Model file for the job. Use its own axes, mm. Give positions to 0.01 mm unless a question says otherwise; leave off trailing zeros. Loops run counter-clockwise (first coordinate to the right, second up) from the corner with the lowest first, then second, coordinate; pieces in that order, holes last. Notation, with made-up numbers: (72, 29) - (131, 29) arc R29 cw to (131, 61) - close; hole circle Ø8 at (-40, 66.5). An arc over 180 degrees is marked (long way). Use a Markdown table: item, result.
from build123d import *

# Parameters (mm, degrees)
SKETCH1_W               = 65.5
SKETCH1_H               = 80
BOSS_EXTRUDE1_DEPTH     = 5
SKETCH2_W               = 7.499999691
SKETCH2_H               = 80
CUT_EXTRUDE1_DEPTH      = 52.938064076
SKETCH3_R               = 12
SKETCH3_R_2             = 1.65
CUT_EXTRUDE2_DEPTH      = 52.938064076
CUT_EXTRUDE3_DEPTH      = 52.938064076
CUT_EXTRUDE3_DEPTH_BACK = 52.938064076
SKETCH4_R               = 4.025


with BuildPart() as part:
    # Sketch1 → Boss-Extrude1 (new body)
    with BuildSketch(Plane.XY):
        Rectangle(SKETCH1_W, SKETCH1_H)
    extrude(amount=BOSS_EXTRUDE1_DEPTH)

    # Sketch2 → Cut-Extrude1 (cut, through all)
    with BuildSketch(Plane.XY.offset(5)):
        with Locations((29.000000155, 0)):
            Rectangle(SKETCH2_W, SKETCH2_H)
    extrude(amount=-CUT_EXTRUDE1_DEPTH, mode=Mode.SUBTRACT)

    # Sketch3 → Cut-Extrude2 (cut, through all)
    with BuildSketch(Plane(origin=(0, 0, 0), x_dir=(-1, 0, 0), z_dir=(0, 0, -1))):
        with Locations((-1.25, 0)):
            Circle(SKETCH3_R)
        with Locations((-16.75, 15.5)):
            Circle(SKETCH3_R_2)
        with Locations((14.25, 15.5)):
            Circle(SKETCH3_R_2)
        with Locations((14.25, -15.5)):
            Circle(SKETCH3_R_2)
        with Locations((-16.75, -15.5)):
            Circle(SKETCH3_R_2)
    extrude(amount=-CUT_EXTRUDE2_DEPTH, mode=Mode.SUBTRACT)

    # Sketch4 → Cut-Extrude3 (cut, two sides: drawn at the far end of the back side and taken through both)
    with BuildSketch(Plane(origin=(0, 0, 0), x_dir=(-1, 0, 0), z_dir=(0, 0, -1)).offset(-CUT_EXTRUDE3_DEPTH_BACK)):
        with Locations((-1.25, 30)):
            Circle(SKETCH4_R)
        with Locations(Location((-1.25, -30, 0), (0, 0, 180))):
            Circle(SKETCH4_R)
    extrude(amount=CUT_EXTRUDE3_DEPTH + CUT_EXTRUDE3_DEPTH_BACK, mode=Mode.SUBTRACT)


solid = part.part
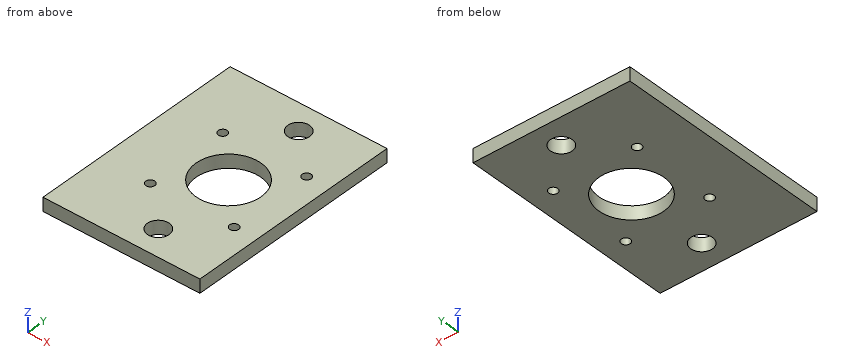
(1) Slice it at B-B, the plane y = 0. Write the cut outline in (x, z).
Computed:
| item | result |
|---|---|
| outline | (-32.75, 0) - (-10.75, 0) - (-10.75, 5) - (-32.75, 5) - close; (13.25, 0) - (25.25, 0) - (25.25, 5) - (13.25, 5) - close |
(2) Drill centre lines: probe 1 along Y at (x, z) = (-14.5, 3.75); probe 2 along Y at (x, z) = (1.25, 3.85) (3 decimals); probe 3 along X at (y, z) = (30, 2) (3 decimals). Where is each one in solid material? Low to high. Write a range as [from, to].
Computed:
| item | result |
|---|---|
| probe 1 | [-40, -17.13], [-13.87, 13.87], [17.13, 40] |
| probe 2 | [-40, -34.025], [-25.975, -12], [12, 25.975], [34.025, 40] |
| probe 3 | [-32.75, -2.775], [5.275, 25.25] |
(3) Slice it at A-A, the plane x = 1.25. Write the cut outline in (y, z) (3 decimals), plus the area to 4 significant figures.
Computed:
| item | result |
|---|---|
| outline | (-40, 0) - (-34.025, 0) - (-34.025, 5) - (-40, 5) - close; (-25.975, 0) - (-12, 0) - (-12, 5) - (-25.975, 5) - close; (12, 0) - (25.975, 0) - (25.975, 5) - (12, 5) - close; (34.025, 0) - (40, 0) - (40, 5) - (34.025, 5) - close |
| area | 199.5 mm² |
(4) Slice it at D-D, the plane x = -9. Write the cut outline in (y, z), plus the area to 3 significant figures.
Computed:
| item | result |
|---|---|
| outline | (-40, 0) - (-6.24, 0) - (-6.24, 5) - (-40, 5) - close; (6.24, 0) - (40, 0) - (40, 5) - (6.24, 5) - close |
| area | 338 mm² |
(5) Pin check, flat tip, straight feed: P1, Ø3, axis at x = 16.75, y = -15.5, coming from the +Z side. Stop position of the tip, or through.
Computed:
| item | result |
|---|---|
| P1 | through |
(6) Slice it at C-C, the plane z = 2.85. Write the cut outline in (x, y) (3 decimals).
Computed:
| item | result |
|---|---|
| outline | (-32.75, -40) - (25.25, -40) - (25.25, 40) - (-32.75, 40) - close; hole circle Ø3.3 at (-14.25, -15.5); hole circle Ø3.3 at (-14.25, 15.5); hole circle Ø24 at (1.25, 0); hole circle Ø8.05 at (1.25, -30); hole circle Ø8.05 at (1.25, 30); hole circle Ø3.3 at (16.75, -15.5); hole circle Ø3.3 at (16.75, 15.5) |
